Read the model definition and answer for the solid it produces. Units are mm, in the model's axes. A direction names the side the tool comes from. Coordinates: 2 decimals unless noted, no trailing zeros. Loops run counter-clockwise (first coordinate to the right, second up) from the corner with the lowest first, then second, coordinate; pieces in that order, holes last. Notation, with made-up numbers: M -16.5,-26.75 L 6.5,-26.75 A24 ccw 6.5,-16.75 Z; hole C 65.25,53 d10. An arc over 180 degrees is marked long. One line per item, written item: value. Start each with the question number.
```python
from build123d import *

# Parameters (mm, degrees)
CYLINDER_R     = 1.6
CYLINDER_DEPTH = 10
BOX001_W       = 61
BOX001_H       = 15
BOX001_DEPTH   = 2
BOX_W          = 82.5
BOX_H          = 15
BOX_DEPTH      = 2


with BuildPart() as taladro1:
    # Cylinder → Cylinder (new body)
    with BuildSketch(Plane(origin=(0, 1.2, -10), x_dir=(1, 0, 0), z_dir=(0, 0, 1))):
        Circle(CYLINDER_R)
    extrude(amount=CYLINDER_DEPTH)


with BuildPart() as perfora_2mm_centro:
    # Box001 → Box001 (new body)
    with BuildSketch(Plane(origin=(12, 0, -2), x_dir=(1, 0, 0), z_dir=(0, 0, 1))):
        with Locations((30.5, 7.5)):
            Rectangle(BOX001_W, BOX001_H)
    extrude(amount=BOX001_DEPTH)


with BuildPart() as fusion001:
    # Box → Box (new body)
    with BuildSketch(Plane.XY):
        with Locations((41.25, 7.5)):
            Rectangle(BOX_W, BOX_H)
    extrude(amount=BOX_DEPTH)

    # Fusion: union perfora_2mm_centro
    add(perfora_2mm_centro.part)


with BuildPart() as fusion001_1:
    # Fusion placement: moved
    add(fusion001.part.moved(Location((-3, -11, -2))))

    # Fusion001: union taladro1
    add(taladro1.part)


with BuildPart() as fusion005:
    # Fusion005 base: copy of taladro1
    add(taladro1.part)

    # Fusion005: union Fusion001
    add(fusion001_1.part)


solid = fusion005.part
```
1) Flat-ended cylindrical pins translate along their axes: pin 1 (7.5 mm diameter, centred on x = 50.5, y = -5.5, fed in from -Z); pin 2 (6 mm diameter, centred on y = -2, z = -5.5, fed in from -X); pin 3 (1.5 mm diameter, centred on y = -6, z = -6.5, fed in from -X); pin 4 (1.5 mm diameter, centred on y = 0, z = -4.5, fed in from +X). Find the tip coordinate at first contact, or state that the pin passes through.
2) A tool of negligible diameter and unlimited length cuts with its end or side. For faces 5 (the face through (-0.208, 2.786, -6.056)), 6 (the face through (0, 1, -10)), 7 (the face through (75, -3, -2)), from which of +Z, -Z, +X, -X, +Y, -Y can it reach the whole face along a straight path? Write none if from no direction.
3) Consider line 1 along Z through (x, y) = (52, -7.25); line 2 along Z through (x, y) = (6, 2); line 3 along X through (y, z) = (-0.25, -5.5). Determine where each line is inside the solid, lowest interval first.
4) Section B-B (y = 1.2) is taken. Determine the outline of the cut face in (x, z).
5) Section D-D (y = -6.25) is taken. Determine the outline of the cut face in (x, z).
6) Section A-A (x = 0) is taken. Determine the outline of the cut face in (y, z).
7) For a pull along X with two mould halves and no side action, classify faces 1 (the face through (-3, -4, -1)), 2 (the face through (9, -4, -3)), 3 (the face through (70, -4, -3)), 4 (the face through (39, -3, -4)) as released by +X, released by -X, zero draft, split by the parting line, or undercut.
8) Section C-C (z = -5) is taken. Determine the outline of the cut face in (x, y).
Results found:
1. pin 1: stops at z = -4
1. pin 2: stops at x = -1.59
1. pin 3: passes through
1. pin 4: stops at x = 70
2. face 5: -Z
2. face 6: -Z, +X, -X, +Y, -Y
2. face 7: -Z, +X, +Y, -Y
3. line 1: z = -4 to 0
3. line 2: z = -2 to 0
3. line 3: x = -0.68 to 0.68
4. outline: M -3,-2 L -1.6,-2 L -1.6,-10 L 1.6,-10 L 1.6,-2 L 9,-2 L 9,-4 L 70,-4 L 70,-2 L 79.5,-2 L 79.5,0 L -3,0 Z
5. outline: M -3,-2 L 9,-2 L 9,-4 L 70,-4 L 70,-2 L 79.5,-2 L 79.5,0 L -3,0 Z
6. outline: M -11,-2 L -0.4,-2 L -0.4,-10 L 2.8,-10 L 2.8,-2 L 4,-2 L 4,0 L -11,0 Z
7. face 1: released by -X
7. face 2: undercut
7. face 3: released by +X
7. face 4: zero draft
8. outline: C 0,1.2 d3.2
